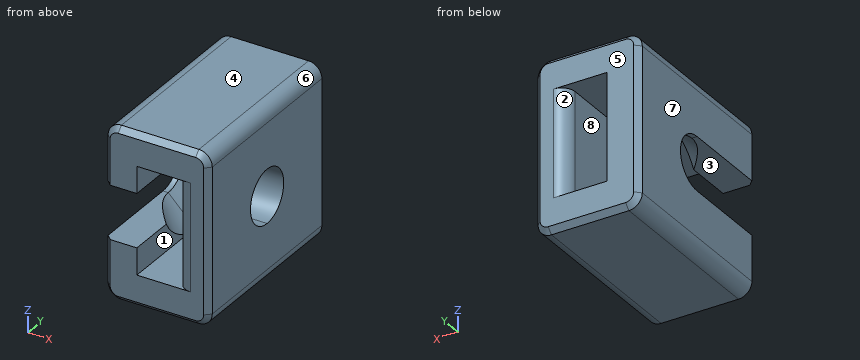
from build123d import *

# Parameters (mm, degrees)
F0_W     = 7.8
F0_H     = 12.8
F0_W_2   = 3
F0_H_2   = 8
F1_DEPTH = 14
F3_DEPTH = 7.801
F4_SIZE  = 1.99999
F5_R     = 1
F6_SIZE  = 0.4
F7_R     = 1
F8_DEPTH = 2.4


# Not quite as in the source:
# - a fillet or chamfer is up to 0.001 mm smaller than in the source, because OpenCascade refuses the exact size


with BuildPart() as f1:
    # F0 (on Front) → F1 (new body)
    with BuildSketch(Plane.XZ):
        Rectangle(F0_W, F0_H)
        Rectangle(F0_W_2, F0_H_2, mode=Mode.SUBTRACT)
    extrude(amount=F1_DEPTH)

    # F2 (on face) → F3 (cut, through all)
    with BuildSketch(Plane(origin=(-3.9, 0, 0), x_dir=(0, -1, 0), z_dir=(-1, 0, 0))):
        with BuildLine():
            Line((7, -2), (7, 2))
            ThreePointArc((7, 2), (5, 0), (7, -2))
        make_face()
        with BuildLine():
            ThreePointArc((7, -2), (8.4142135624, -1.4142135624), (9, 0))
            ThreePointArc((9, 0), (8.4142135624, 1.4142135624), (7, 2))
            Line((7, 2), (7, -2))
        make_face()
    extrude(amount=-F3_DEPTH, mode=Mode.SUBTRACT)

    # F4 (size 2 in the source; OpenCascade refuses exactly that, so slightly less here)
    f4_edges = [f1.edges().sort_by_distance(p)[0] for p in [
        (-1.5, -7, 2),
    ]]
    chamfer(f4_edges, length=F4_SIZE)

    # F5
    f5_edges = [f1.edges().sort_by_distance(p)[0] for p in [
        (3.9, -7, 6.4),
        (3.9, -7, -6.4),
        (-3.9, -7, -6.4),
        (-3.9, -7, 6.4),
    ]]
    fillet(f5_edges, radius=F5_R)

    # F6
    f6_edges = [f1.edges().sort_by_distance(p)[0] for p in [
        (3.9, -14, 0),
        (3.9, 0, 0),
    ]]
    chamfer(f6_edges, length=F6_SIZE)

    # F7
    f7_edges = [f1.edges().sort_by_distance(p)[0] for p in [
        (1.5, -14, 0),
        (1.5, 0, 0),
    ]]
    fillet(f7_edges, radius=F7_R)

    # F2 (on face) → F8 (cut, through all)
    with BuildSketch(Plane(origin=(-3.9, 0, 0), x_dir=(0, -1, 0), z_dir=(-1, 0, 0))):
        with BuildLine():
            ThreePointArc((7, 2), (8.4142135624, 1.4142135624), (9, 0))
            ThreePointArc((9, 0), (8.4142135624, -1.4142135624), (7, -2))
            Line((7, -2), (14, -2))
            Line((14, -2), (14, 2))
            Line((14, 2), (7, 2))
        make_face()
    extrude(amount=-F8_DEPTH, mode=Mode.SUBTRACT)


solid = f1.part
Input: part model. Units: mm. Frame: model coordinates. Face numbers are marked on the shaded views. A direction names the side the tool comes from. Round coordinates to 2 decimals unless told otherwise and drop trailing zeros. Write each loop counter-clockwise with the first axis right and the second up, starting at its lowest first coordinate (ties: lowest second). Pieces come first, ordered by that corner, then holes.
1) Draft query along X for the marked faces 6, 7 and 8. Return one class per face: pulls with the +X half, pulls with the -X half, needs draft (parallel to the pull), parting line crosses it, or undercut.
2) Contact query for a flat-ended pin moving along its axis: P1, Ø2, axis at x = 0, z = 1.5, coming from the -Y side. Output: stop coordinate, or through.
3) Cut plane C-C (x = 2). Return the cut outline in (y, z).
4) Cut plane B-B (y = -2.75). Return the cut outline in (x, z).
5) Cut plane D-D (z = -1). Count the separate pieces of the cut face and the enclosed holes in it, then the cut area to 3 significant figures.
6) Ray query, L1, parallel to Z at x = 1, y = -12.25; L2, parallel to X at y = -13, z = 3.25; L3, parallel to Z at x = 1.75, y = -8. Return the intervals inside material, ascending.
7) Reachability of the marked faces 1, 2, 3, 4 and 5 from +Z, -Z, +X, -X, +Y, -Y: full face, straight path, thin tool, end or side. Return the list, or none.
8) Cut plane A-A (x = -0.5). Return the cut outline in (y, z).
Geometry says:
1. face 6: pulls with the +X half
1. face 7: pulls with the -X half
1. face 8: undercut
2. P1: passes through
3. outline: (-14, -6) - (-13.6, -6.4) - (-0.4, -6.4) - (0, -6) - (0, -4) - (-0.13, -4) - (-0.13, 4) - (0, 4) - (0, 6) - (-0.4, 6.4) - (-13.6, 6.4) - (-14, 6) - (-14, 4) - (-13.87, 4) - (-13.87, -4) - (-14, -4) - close; hole circle Ø4 at (-7, 0)
4. outline: (-3.9, -5.4) arc R1 ccw to (-2.9, -6.4) - (2.9, -6.4) arc R1 ccw to (3.9, -5.4) - (3.9, 5.4) arc R1 ccw to (2.9, 6.4) - (-2.9, 6.4) arc R1 ccw to (-3.9, 5.4) - close; hole (-1.5, -4) - (1.5, -4) - (1.5, 4) - (-1.5, 4) - close
5. separate pieces: 3
5. enclosed holes: 0
5. area: 35.1 mm2
6. L1: z = -6.4 to -4, 4 to 6.4
6. L2: x = -3.9 to -1.5, 1.5 to 3.9
6. L3: z = -6.4 to -1.73, 1.73 to 6.4
7. face 1: +Y, -Y
7. face 2: +Y
7. face 3: -X, -Y
7. face 4: +Z, +X, -X, +Y, -Y
7. face 5: +Z, -Z, +X, -X, +Y
8. outline: (-14, -6) - (-13.6, -6.4) - (-0.4, -6.4) - (0, -6) - (0, -4) - (-14, -4) - close; (-14, 4) - (0, 4) - (0, 6) - (-0.4, 6.4) - (-13.6, 6.4) - (-14, 6) - close
